```python
from build123d import *

# Parameters (mm, degrees)
BOSS_EXTRUDE1_DEPTH = 17
SKETCH3_R           = 6
CUT_EXTRUDE1_DEPTH  = 10
SKETCH4_OUTSIDE_W   = 536.486
SKETCH4_OUTSIDE_H   = 479.866
CUT_EXTRUDE2_DEPTH  = 8
SKETCH5_R           = 1.25
CUT_EXTRUDE3_DEPTH  = 281.053566305
SKETCH7_R           = 1.25
CUT_EXTRUDE5_DEPTH  = 281.053566305
CUT_EXTRUDE6_DEPTH  = 281.053566305
SKETCH9_R           = 1
CUT_EXTRUDE7_DEPTH  = 270.381390102


with BuildPart() as part:
    # Sketch1 → Boss-Extrude1 (new body)
    with BuildSketch(Plane.XY):
        Polygon((105.655099262, 183), (-105.655099262, 183), (-211.310198523, 0), (-105.655099262, -183), (105.655099262, -183), (211.310198523, 0), align=None)
    extrude(amount=BOSS_EXTRUDE1_DEPTH)

    # Sketch3 → Cut-Extrude1 (cut)
    with BuildSketch(Plane.XY.offset(17)):
        with Locations((50, 147)):
            Circle(SKETCH3_R)
        with Locations((-50, 147)):
            Circle(SKETCH3_R)
        with Locations((-152.305734356, -30.198729811)):
            Circle(SKETCH3_R)
        with Locations((-102.305734356, -116.801270189)):
            Circle(SKETCH3_R)
        with Locations((102.305734356, -116.801270189)):
            Circle(SKETCH3_R)
        with Locations((152.305734356, -30.198729811)):
            Circle(SKETCH3_R)
    extrude(amount=-CUT_EXTRUDE1_DEPTH, mode=Mode.SUBTRACT)

    # Sketch4 outside → Cut-Extrude2 (cut)
    with BuildSketch(Plane.XY.offset(17)):
        Rectangle(SKETCH4_OUTSIDE_W, SKETCH4_OUTSIDE_H)
        Polygon((191.680289371, 0), (95.840144685, 166), (-95.840144685, 166), (-191.680289371, 0), (-95.840144685, -166), (95.840144685, -166), align=None, mode=Mode.SUBTRACT)
    extrude(amount=-CUT_EXTRUDE2_DEPTH, mode=Mode.SUBTRACT)

    # Sketch5 → Cut-Extrude3 (cut, through all)
    with BuildSketch(Plane.XY.offset(17)):
        with Locations((115.181378703, -66.5)):
            Circle(SKETCH5_R)
        with Locations((97.860870628, -56.5)):
            Circle(SKETCH5_R)
        with Locations((-115.181378703, -66.5)):
            Circle(SKETCH5_R)
        with Locations((-97.860870628, -56.5)):
            Circle(SKETCH5_R)
        with Locations((0, 133)):
            Circle(SKETCH5_R)
        with Locations((0, 113)):
            Circle(SKETCH5_R)
        with BuildLine():
            Line((-121.194518424, -67.084936491), (-118.694518424, -71.415063509))
            ThreePointArc((-118.694518424, -71.415063509), (-119.609581934, -74.830127019), (-123.024645443, -73.915063509))
            Line((-123.024645443, -73.915063509), (-125.524645443, -69.584936491))
            ThreePointArc((-125.524645443, -69.584936491), (-124.609581934, -66.169872981), (-121.194518424, -67.084936491))
        make_face()
        with BuildLine():
            Line((-131.58682327, -73.084936491), (-129.08682327, -77.415063509))
            ThreePointArc((-129.08682327, -77.415063509), (-130.001886779, -80.830127019), (-133.416950288, -79.915063509))
            Line((-133.416950288, -79.915063509), (-135.916950288, -75.584936491))
            ThreePointArc((-135.916950288, -75.584936491), (-135.001886779, -72.169872981), (-131.58682327, -73.084936491))
        make_face()
        with BuildLine():
            Line((118.694518424, -71.415063509), (121.194518424, -67.084936491))
            ThreePointArc((121.194518424, -67.084936491), (124.609581934, -66.169872981), (125.524645443, -69.584936491))
            Line((125.524645443, -69.584936491), (123.024645443, -73.915063509))
            ThreePointArc((123.024645443, -73.915063509), (119.609581934, -74.830127019), (118.694518424, -71.415063509))
        make_face()
        with BuildLine():
            Line((129.08682327, -77.415063509), (131.58682327, -73.084936491))
            ThreePointArc((131.58682327, -73.084936491), (135.001886779, -72.169872981), (135.916950288, -75.584936491))
            Line((135.916950288, -75.584936491), (133.416950288, -79.915063509))
            ThreePointArc((133.416950288, -79.915063509), (130.001886779, -80.830127019), (129.08682327, -77.415063509))
        make_face()
        with BuildLine():
            Line((2.5, 138.5), (-2.5, 138.5))
            ThreePointArc((-2.5, 138.5), (-5, 141), (-2.5, 143.5))
            Line((-2.5, 143.5), (2.5, 143.5))
            ThreePointArc((2.5, 143.5), (5, 141), (2.5, 138.5))
        make_face()
        with BuildLine():
            Line((2.5, 150.5), (-2.5, 150.5))
            ThreePointArc((-2.5, 150.5), (-5, 153), (-2.5, 155.5))
            Line((-2.5, 155.5), (2.5, 155.5))
            ThreePointArc((2.5, 155.5), (5, 153), (2.5, 150.5))
        make_face()
    extrude(amount=-CUT_EXTRUDE3_DEPTH, mode=Mode.SUBTRACT)

    # Sketch7 → Cut-Extrude5 (cut, through all)
    with BuildSketch(Plane(origin=(0, 0, 0), x_dir=(-1, 0, 0), z_dir=(0, 0, -1))):
        with Locations((147.640670847, 33.27885683)):
            Circle(SKETCH7_R)
        with Locations((102.640670847, 111.22114317)):
            Circle(SKETCH7_R)
        with Locations((45, -144.5)):
            Circle(SKETCH7_R)
        with Locations((-45, -144.5)):
            Circle(SKETCH7_R)
        with Locations((-147.640670847, 33.27885683)):
            Circle(SKETCH7_R)
        with Locations((-102.640670847, 111.22114317)):
            Circle(SKETCH7_R)
    extrude(amount=-CUT_EXTRUDE5_DEPTH, mode=Mode.SUBTRACT)

    # Sketch8 → Cut-Extrude6 (cut, through all)
    with BuildSketch(Plane(origin=(0, 0, 0), x_dir=(-1, 0, 0), z_dir=(0, 0, -1))):
        Polygon((105.655099262, 183), (-105.655099262, 183), (-211.310198523, 0), (-105.655099262, -183), (105.655099262, -183), (211.310198523, 0), align=None)
        Polygon((101.613647377, 176), (-101.613647377, 176), (-203.227294755, 0), (-101.613647377, -176), (101.613647377, -176), (203.227294755, 0), align=None, mode=Mode.SUBTRACT)
    extrude(amount=-CUT_EXTRUDE6_DEPTH, mode=Mode.SUBTRACT)

    # Sketch9 → Cut-Extrude7 (cut, through all)
    with BuildSketch(Plane(origin=(0, 0, 0), x_dir=(-1, 0, 0), z_dir=(0, 0, -1))):
        with Locations((-118.35021945, 137.610699371)):
            Circle(SKETCH9_R)
        with Locations((-178.349471213, 33.688946902)):
            Circle(SKETCH9_R)
        with Locations((-178.090344047, -33.538475773)):
            Circle(SKETCH9_R)
        with Locations((-118.090344047, -137.461524227)):
            Circle(SKETCH9_R)
        with Locations((-60, -171)):
            Circle(SKETCH9_R)
        with Locations((60, -171)):
            Circle(SKETCH9_R)
        with Locations((118.35021945, -137.610699371)):
            Circle(SKETCH9_R)
        with Locations((178.349471213, -33.688946902)):
            Circle(SKETCH9_R)
        with Locations(Location((60, 171, 0), (0, 0, 180))):
            Circle(SKETCH9_R)
        with Locations(Location((-60, 171, 0), (0, 0, 180))):
            Circle(SKETCH9_R)
    extrude(amount=-CUT_EXTRUDE7_DEPTH, mode=Mode.SUBTRACT)


solid = part.part
```
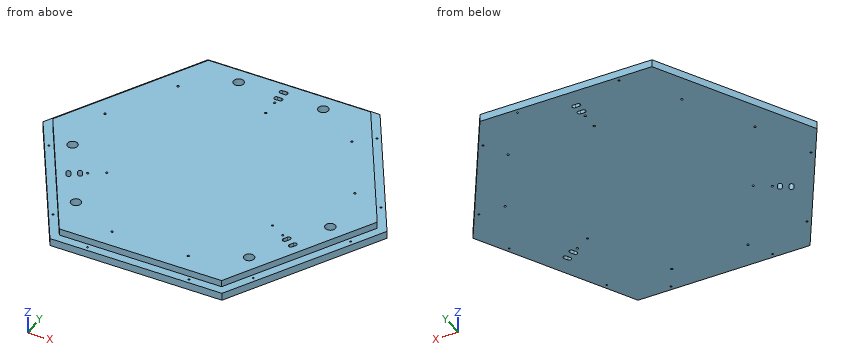
The model under review builds one solid part; all positions refer to its coordinate system, in mm. Give positions to 0.01 mm unless a question says otherwise; leave off trailing zeros. Write each loop counter-clockwise with the first axis right and the second up, starting at its lowest first coordinate (ties: lowest second). Pieces come first, ordered by that corner, then holes. Notation, with made-up numbers: (37.5, -35) -> (73.5, -35) arc R29 ccw to (73.5, -14) -> close; hole circle Ø9 at (-20.5, 39). An arc over 180 degrees is marked (long way). Put each result on its own line as item: value.
(1) We need section A-A, the plane x = -88. Give the boundary of the cut face in (y, z), and give its area (3 significant figures).
Results are:
outline: (-176, 0) -> (176, 0) -> (176, 9) -> (166, 9) -> (166, 17) -> (-166, 17) -> (-166, 9) -> (-176, 9) -> close
area: 5,820 mm²
(2) For pin 1 Ø9.5 at (x, y) = (102.31, -116.8) entering from +Z; pin 2 Ø1 at (y, z) = (104, 2) entering from -X; pin 3 Ø2 at (x, z) = (143.5, 2.5) entering from -Y, all flat-tipped, find the tip position at first contact; note any pin that passes through.
Results are:
pin 1: z = 7
pin 2: x = -143.47
pin 3: y = -105.18
(3) To check wall thickness, follow probe 1 along Y at (x, z) = (60, 5.75); probe 2 along X at (y, z) = (-26, 12.75); probe 3 along X at (y, z) = (-116, 12.75). State the ranges of each line that lie inside material, in increasing order. Write a range as from..to.
Results are:
probe 1: -176..-172, -170..170, 172..176
probe 2: -176.67..-156.59, -148.02..148.02, 156.59..176.67
probe 3: -124.71..-108.25, -96.36..96.36, 108.25..124.71
(4) We need section B-B, the plane y = 47. Give the boundary of the cut face in (x, z), and give its area (3 significant figures).
Results are:
outline: (-176.09, 0) -> (176.09, 0) -> (176.09, 9) -> (164.54, 9) -> (164.54, 17) -> (-164.54, 17) -> (-164.54, 9) -> (-176.09, 9) -> close
area: 5,800 mm²
(5) We need section C-C, the plane z = 3.25. State how many separate pieces and enclosed holes the cut face has, and give its area (3 significant figures).
Results are:
separate pieces: 1
enclosed holes: 28
area: 107,000 mm²
